from build123d import *

# Parameters (mm, degrees)
F1_DEPTH  = 2.1
F3_DEPTH  = 20
F5_DEPTH  = 2.1
F6_R      = 5
F8_DEPTH  = 2
F11_DEPTH = 2


with BuildPart() as f1:
    # F0 (on Top) → F1 (new body)
    with BuildSketch(Plane.XY):
        with BuildLine():
            Line((-15, 0), (0, 0))
            Line((0, 0), (0, 35))
            Line((0, 35), (-15, 35))
            ThreePointArc((-15, 35), (-18.5355339059, 33.5355339059), (-20, 30))
            Line((-20, 30), (-20, 5))
            ThreePointArc((-20, 5), (-18.5355339059, 1.4644660941), (-15, 0))
        make_face()
        with BuildLine():
            ThreePointArc((-12.1489869425, 27.9340066588), (-10.0330005573, 30.1497467207), (-7.85, 27.9999999982))
            Line((-7.85, 27.9999999982), (-7.8500000178, 7))
            ThreePointArc((-7.8500000178, 7), (-10.0000000178, 4.85), (-12.1500000178, 7))
            ThreePointArc((-12.1500000178, 7), (-12.1500000172, 7.0000520234), (-12.1500000153, 7.0001040468))
            Line((-12.1500000153, 7.0001040468), (-12.1489869425, 27.9340066588))
        make_face(mode=Mode.SUBTRACT)
    extrude(amount=F1_DEPTH)

    # F2 (on Top) → F3 (join)
    with BuildSketch(Plane.XY):
        Polygon((0, 35), (0, 0.0720546025), (2.1, 0), (2.1, 35), align=None)
    extrude(amount=F3_DEPTH)

    # F4 (on Right) → F5 (cut, through all)
    with BuildSketch(Plane.YZ):
        with BuildLine():
            Line((9.25, 5), (9.25, 15))
            ThreePointArc((9.25, 15), (7, 17.25), (4.75, 15))
            ThreePointArc((4.75, 15), (4.7500000019, 14.9999071898), (4.7500000077, 14.9998143795))
            Line((4.7500000077, 14.9998143795), (4.7508199613, 5.0607384035))
            Line((4.7508199613, 5.0607384035), (4.7508300135, 4.9388904917))
            ThreePointArc((4.7508300135, 4.9388904917), (7.0305575724, 2.750207513), (9.25, 5))
        make_face()
        with BuildLine():
            ThreePointArc((4.7508199613, 5.0607384035), (4.7500000077, 4.9998143795), (4.7508300135, 4.9388904917))
            Line((4.7508300135, 4.9388904917), (4.7508199613, 5.0607384035))
        make_face()
        with BuildLine():
            ThreePointArc((25.75, 5), (27.9694424276, 2.750207513), (30.2491699865, 4.9388904917))
            Line((30.2491699865, 4.9388904917), (30.2491800387, 5.0607384035))
            Line((30.2491800387, 5.0607384035), (30.2499999923, 14.9998143795))
            Line((30.2499999923, 14.9998143795), (30.2500000077, 15))
            ThreePointArc((30.25, 15), (28, 17.25), (25.75, 15))
            Line((25.75, 15), (25.75, 5))
        make_face()
        with BuildLine():
            Line((30.2491800387, 5.0607384035), (30.2491699865, 4.9388904917))
            ThreePointArc((30.2491699865, 4.9388904917), (30.2499999923, 4.9998143795), (30.2491800387, 5.0607384035))
        make_face()
    extrude(amount=F5_DEPTH, mode=Mode.SUBTRACT)

    # F6
    f6_edges = [f1.edges().sort_by_distance(p)[0] for p in [
        (1.05, 35, 20),
        (1.05, 0.036027, 20),
    ]]
    fillet(f6_edges, radius=F6_R)

    # F7 (on Front) → F8 (join)
    with BuildSketch(Plane.XZ):
        Polygon((-7, 2.1), (0, 2.1), (0, 9.1), align=None)
    extrude(amount=-F8_DEPTH)

    # F10 (on offset) → F11 (join)
    with BuildSketch(Plane(origin=(0, 35, 0), x_dir=(-1, 0, 0), z_dir=(0, 1, 0))):
        Polygon((0, 9.1), (0, 2.1), (7, 2.1), align=None)
    extrude(amount=-F11_DEPTH)


solid = f1.part
Check sheet for the modelled part. Datum: model origin and axes. Units: mm. A direction names the side the tool comes from. Give positions to 0.01 mm unless a question says otherwise; leave off trailing zeros. Loops run counter-clockwise (first coordinate to the right, second up) from the corner with the lowest first, then second, coordinate; pieces in that order, holes last. Notation, with made-up numbers: M 26,73.5 L 49,73.5 A17 ccw 49,83.5 Z; hole C 6,32.5 d8. An arc over 180 degrees is marked long. Return JSON: item names as keys, results as strings. Group by question number.
1. Mould release check, pull along Z, two halves, no side actions. Record for faces 1 (the cylindrical face through (-10.08, 30.15, 1.04)), 2 (the flat face through (1, 9.25, 10)), 3 (the cylindrical face through (1.029, 1.463, 18.496)): released by +Z, released by -Z, zero draft, split by the parting line, or undercut.
2. Tool access check on faces 4 (the flat face through (-7.85, 18, 1)), 5 (the flat face through (1, 18, 20)), 6 (the flat face through (-7, 18, 0)), 7 (the cylindrical face through (1.04, 7.05, 17.25)), 8 (the flat face through (-2, 2, 4)). Record the directions out of +Z, -Z, +X, -X, +Y, -Y that give a thin tool (end or side, any length) a straight path to the whole face; none if there is none.
3. Cross-section at C-C on z = 4. Record the boundary of the cut face in (x, y), plus the area to 3 significant figures.
4. Cross-section at A-A on x = -10. Record the boundary of the cut face in (y, z), plus the area to 3 significant figures.
5. Cross-section at D-D on x = -5. Record the boundary of the cut face in (y, z), plus the area to 3 significant figures.
6. Thickness scan on L1, parallel to Z at x = -4.25, y = 26; L2, parallel to Y at x = -1.5, z = 4.75. Record the ranges inside material, lowest first.
7. Go/stop test with flat-tipped pins: pin 1 (3 mm diameter, centred on x = -0.5, y = 17, fed in from -Z); pin 2 (1.7 mm diameter, centred on x = 1, z = 7.5, fed in from -Y); pin 3 (2 mm diameter, centred on x = -17.5, y = 27.5, fed in from +Z); pin 4 (5.5 mm diameter, centred on y = 12.5, z = 15, fed in from -X). Record where each tip stops, or that it passes through.
8. Cross-section at B-B on y = 24.5. Record the boundary of the cut face in (x, z), plus the area to 3 significant figures.
Return value:
{
 "1": {"face 1": "zero draft", "face 2": "undercut", "face 3": "released by +Z"},
 "2": {"face 4": "+Z, -Z", "face 5": "+Z, +X, -X, +Y, -Y", "face 6": "-Z, +X, -X, +Y, -Y", "face 7": "+X, -X", "face 8": "+Z, -X"},
 "3": {"outline": "M -5.1,0 L 0,0 L 0,0.07 L 2.1,0 L 2.1,4.98 L 0,4.98 L 0,2 L -5.1,2 Z; M -5.1,33 L 0,33 L 0,30.02 L 2.1,30.02 L 2.1,35 L -5.1,35 Z; M 0,9.02 L 2.1,9.02 L 2.1,25.98 L 0,25.98 Z", "area": "76.9 mm^2"},
 "4": {"outline": "M 0,0 L 4.85,0 L 4.85,2.1 L 0,2.1 Z; M 30.15,0 L 35,0 L 35,2.1 L 30.15,2.1 Z", "area": "20.4 mm^2"},
 "5": {"outline": "M 0,0 L 35,0 L 35,4.1 L 33,4.1 L 33,2.1 L 2,2.1 L 2,4.1 L 0,4.1 Z", "area": "81.5 mm^2"},
 "6": {"L1": "0 to 2.1", "L2": "0 to 2, 33 to 35"},
 "7": {"pin 1": "z = 0", "pin 2": "y = 0.01", "pin 3": "z = 2.1", "pin 4": "x = 0"},
 "8": {"outline": "M -20,0 L -12.15,0 L -12.15,2.1 L -20,2.1 Z; M -7.85,0 L 2.1,0 L 2.1,20 L 0,20 L 0,2.1 L -7.85,2.1 Z", "area": "75.0 mm^2"}
}
